Autodesk Fusion 360 part; units mm, degrees
sketch "Sketch1" plane through (0, 0, 0) normal (0, 0, 1) x (1, 0, 0)
  line L0 (0, 0) -> (131, 0)
  line L1 (131, 0) -> (131, 36.5)
  line L2 (131, 36.5) -> (0, 36.5)
  line L3 (0, 36.5) -> (0, 0)
  line L4 (65.5, 18.25) -> (96.5, 18.25)
  line L5 (65.5, 18.25) -> (34.5, 18.25)
  circle A0 centre (34.5, 18.25) radius 12
  circle A1 centre (96.5, 18.25) radius 12
  circle A2 centre (34.5, 18.25) radius 10
  circle A3 centre (96.5, 18.25) radius 10
  circle A4 centre (34.5, 18.25) radius 6.5
  circle A5 centre (96.5, 18.25) radius 6.5
  circle A6 centre (34.5, 18.25) radius 2
  circle A7 centre (96.5, 18.25) radius 2
  dimension "d1" = 131
  dimension "d2" = 36.5
  dimension "d3" = 31
  dimension "d4" = 31
  dimension "d5" = 24
  dimension "d6" = 24
  dimension "d7" = 20
  dimension "d8" = 20
  dimension "d9" = 13
  dimension "d10" = 13
  dimension "d17" = 4
  dimension "d18" = 4
extrude "Extrude1" add sketch "Sketch1" against normal blind 196 contours L0 L1 L2 L3 | A7 | A5 | A3 | A1 | A6 | A4 | A2 | A0
extrude "Extrude2" add sketch "Sketch1" along normal blind 1 contours A1 | A0
extrude "Extrude3" add sketch "Sketch1" along normal blind 4 contours A3 | A2
extrude "Extrude4" add sketch "Sketch1" along normal blind 5 contours A5 | A4
fillet "Fillet1" radius 1 4 edges at (0, 0, -98) (131, 0, -98) (131, 36.5, -98) (0, 36.5, -98) 1 faces at (13.6667, 18.25, -196)
equation "d3 = ( 62 / 2 ) * 1 mm"
equation "d4 = ( 62 / 2 ) * 1 mm"
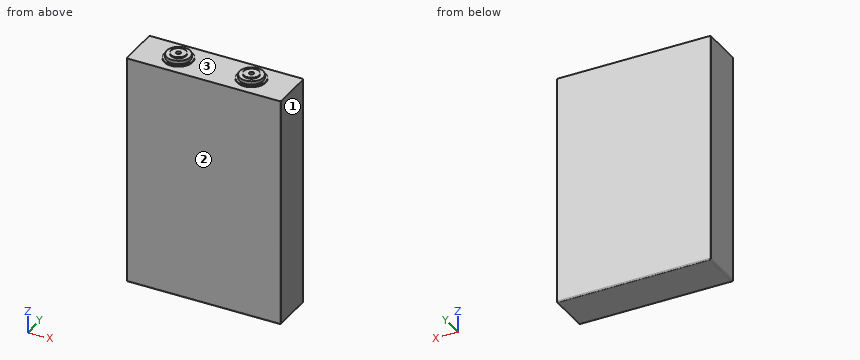
Input: part model. Units: mm. Frame: model coordinates. Face numbers are marked on the shaded views. Round coordinates to 2 decimals unless told otherwise and drop trailing zeros. Loops run counter-clockwise (first coordinate to the right, second up) from the corner with the lowest first, then second, coordinate; pieces in that order, holes last. Notation, with made-up numbers: M 11,44 L 35,44 A18 cw 35,50 Z; hole C -20.5,60 d9. An arc over 180 degrees is marked long. Answer as CSV lines item,"result". Start each with the question number.
(1) Draft query along X for the marked faces 1, 2 and 3. Return one class per face: released by +X, released by -X, zero draft, split by the parting line, or undercut.
(2) Section B-B, the plane x = 64. Output: boundary loops of the cut face in (y, z), plus the area to 3 significant figures.
(3) Line query: line 1 (X direction, y = 18, z = 2); line 2 (Y direction, x = 96.5, z = 3.55); line 3 (Z direction, x = 86, y = 16.5). Output: solid intervals per line, ascending. Write a range as [from, to].
(4) First-contact query: pin 1 (1.2 mm diameter, centred on x = 33.5, y = 19, fed in from +Z). Flat tip, straight axial feed; report the tip coordinate or a pass-through.
(5) Section A-A, the plane y = 33. Output: boundary loops of the cut face in (x, z).
Values found:
1,face 1,"released by +X"
1,face 2,"zero draft"
1,face 3,"undercut"
2,outline,"M 0,-195 A1 ccw 1,-196 L 35.5,-196 A1 ccw 36.5,-195 L 36.5,0 L 0,0 Z"
2,area,"7,150 mm²"
3,line 1,"x = [24.5, 32.52], [36.48, 44.5], [86.5, 94.52], [98.48, 106.5]"
3,line 2,"y = [8.25, 16.25], [20.25, 28.25]"
3,line 3,"z = [-196, 1]"
4,pin 1,"stops at z = 0"
5,outline,"M 0,-195 A1 ccw 1,-196 L 130,-196 A1 ccw 131,-195 L 131,0 L 0,0 Z"
